from build123d import *

# Parameters (mm, degrees)
SKETCH1_W                                           = 159.95
SKETCH1_H                                           = 159.95
BOSS_EXTRUDE2_DEPTH                                 = 30
SKETCH3_W                                           = 7
SKETCH3_H                                           = 10
BOSS_EXTRUDE4_DEPTH                                 = 145.45
CHAMFER1_SIZE                                       = 0.508
CHAMFER1_SIZE2                                      = 0.03552282
CHAMFER2_SIZE                                       = 0.508
CHAMFER2_SIZE2                                      = 0.03552282
SKETCH4_W                                           = 7.1
SKETCH4_H                                           = 10.2
CUT_EXTRUDE6_DEPTH                                  = 160.2
FILLET1_R                                           = 1
SKETCH6_W                                           = 10.35
SKETCH6_H                                           = 14.5
CUT_EXTRUDE7_DEPTH                                  = 80
BOSS_EXTRUDE5_REACH                                 = 206.773
SKETCH7_W                                           = 14.5
SKETCH7_H                                           = 10.25
CSK_FOR_M4_COUNTERSUNK_FLAT_HEAD_SCREW1_D           = 4.5
CSK_FOR_M4_COUNTERSUNK_FLAT_HEAD_SCREW1_DEPTH       = 16
CSK_FOR_M4_COUNTERSUNK_FLAT_HEAD_SCREW1_CSINK_D     = 9.4
CSK_FOR_M4_COUNTERSUNK_FLAT_HEAD_SCREW1_CSINK_ANGLE = 90
CSK_FOR_M4_COUNTERSUNK_FLAT_HEAD_SCREW1_TIP         = 1.351936393
SKETCH12_R                                          = 2.5
CUT_EXTRUDE9_DEPTH                                  = 5
FILLET2_START                                       = -15.571212121
FILLET2_DEPTH                                       = 154.571212121
FILLET3_START                                       = -15.571212121
FILLET3_DEPTH                                       = 154.571212121
M2_TAPPED_HOLE1_D                                   = 1.6
M2_TAPPED_HOLE1_DEPTH                               = 5.2
M2_TAPPED_HOLE1_TIP                                 = 0.480688495
SKETCH29_W                                          = 20.8
SKETCH29_H                                          = 20.8
SKETCH29_W_2                                        = 12.85
SKETCH29_H_2                                        = 12.85
BOSS_EXTRUDE6_DEPTH                                 = 38
CUT_EXTRUDE15_DEPTH                                 = 207.096620322
CUT_EXTRUDE15_DEPTH_BACK                            = 207.096620322
SKETCH26_W                                          = 10
SKETCH26_H                                          = 10
CUT_EXTRUDE16_DEPTH                                 = 8.5
CUT_EXTRUDE16_DEPTH_BACK                            = 98.4
SKETCH30_W                                          = 10
SKETCH30_H                                          = 10
SKETCH31_W                                          = 12.85
SKETCH31_H                                          = 12.85
CUT_EXTRUDE17_DEPTH                                 = 20
FILLET4_R                                           = 1


with BuildPart() as part:
    # Sketch1 → Boss-Extrude2 (new body)
    with BuildSketch(Plane(origin=(0, 0, 0), x_dir=(1, 0, 0), z_dir=(0, 1, 0))):
        with Locations((57.653787879, -61.85)):
            Rectangle(SKETCH1_W, SKETCH1_H)
    extrude(amount=BOSS_EXTRUDE2_DEPTH)

    # Sketch3 → Boss-Extrude4 (add)
    with BuildSketch(Plane.XY.offset(-18.125)):
        with Locations((141.128787879, 15)):
            Rectangle(SKETCH3_W, SKETCH3_H)
    extrude(amount=BOSS_EXTRUDE4_DEPTH)

    # Chamfer1
    chamfer1_edges = [part.edges().sort_by_distance(p)[0] for p in [
        (144.628787879, 20, 54.6),
    ]]
    chamfer1_side = [part.faces().sort_by_distance(p)[0] for p in [
        (141.128787879, 20, 54.6),
    ]]
    chamfer(chamfer1_edges, length=CHAMFER1_SIZE, length2=CHAMFER1_SIZE2, reference=chamfer1_side[0])

    # Chamfer2
    chamfer2_edges = [part.edges().sort_by_distance(p)[0] for p in [
        (144.628787879, 10, 54.6),
    ]]
    chamfer2_side = [part.faces().sort_by_distance(p)[0] for p in [
        (141.128787879, 10, 54.6),
    ]]
    chamfer(chamfer2_edges, length=CHAMFER2_SIZE, length2=CHAMFER2_SIZE2, reference=chamfer2_side[0])

    # Sketch4 → Cut-Extrude6 (cut)
    with BuildSketch(Plane.ZY.offset(-144.628787879)):
        with Locations((-14.575, 15)):
            Rectangle(SKETCH4_W, SKETCH4_H)
    extrude(amount=CUT_EXTRUDE6_DEPTH, mode=Mode.SUBTRACT)

    # Fillet1
    fillet1_edges = [part.edges().sort_by_distance(p)[0] for p in [
        (144.628787879, 15, -11.025),
    ]]
    fillet(fillet1_edges, radius=FILLET1_R)

    # Sketch6 → Cut-Extrude7 (cut)
    with BuildSketch(Plane(origin=(0, 30, 0), x_dir=(1, 0, 0), z_dir=(0, 1, 0))):
        with Locations((132.453787879, -134.575)):
            Rectangle(SKETCH6_W, SKETCH6_H)
    extrude(amount=-CUT_EXTRUDE7_DEPTH, mode=Mode.SUBTRACT)

    # Boss-Extrude5: up to this face of the body (flat: up to its plane)
    boss_extrude5_end = Plane(part.part.faces().sort_by_distance((57.212424271, 0, 61.420880102))[0])
    # Sketch7 → Boss-Extrude5 (add, up to the picked face)
    with BuildSketch(Plane(origin=(0, 30, 0), x_dir=(1, 0, 0), z_dir=(0, 1, 0)), mode=Mode.PRIVATE) as boss_extrude5_sk1:
        with Locations((-15.071212121, 23.25)):
            Rectangle(SKETCH7_W, SKETCH7_H)
    boss_extrude5_tool1 = split(extrude(boss_extrude5_sk1.sketch, amount=-BOSS_EXTRUDE5_REACH, mode=Mode.PRIVATE), bisect_by=boss_extrude5_end, keep=Keep.BOTH, mode=Mode.PRIVATE)
    add(boss_extrude5_tool1.solids().sort_by(Axis((-15.071212, 30, -23.25), (0, -1, 0)))[0])

    # CSK for M4 Countersunk Flat Head Screw1
    with Locations(Plane.ZY.offset(22.321212121)):
        with Locations((-21, 15)):
            CounterSinkHole(CSK_FOR_M4_COUNTERSUNK_FLAT_HEAD_SCREW1_D / 2, CSK_FOR_M4_COUNTERSUNK_FLAT_HEAD_SCREW1_CSINK_D / 2, depth=CSK_FOR_M4_COUNTERSUNK_FLAT_HEAD_SCREW1_DEPTH, counter_sink_angle=CSK_FOR_M4_COUNTERSUNK_FLAT_HEAD_SCREW1_CSINK_ANGLE)
            with Locations((0, 0, -(CSK_FOR_M4_COUNTERSUNK_FLAT_HEAD_SCREW1_DEPTH + CSK_FOR_M4_COUNTERSUNK_FLAT_HEAD_SCREW1_TIP / 2))):  # 118° drill point
                Cone(0, CSK_FOR_M4_COUNTERSUNK_FLAT_HEAD_SCREW1_D / 2, CSK_FOR_M4_COUNTERSUNK_FLAT_HEAD_SCREW1_TIP, mode=Mode.SUBTRACT)

    # Sketch12 → Cut-Extrude9 (cut)
    with BuildSketch(Plane.XY.offset(127.325)):
        with Locations((132.453787879, 15)):
            Circle(SKETCH12_R)
    extrude(amount=-CUT_EXTRUDE9_DEPTH, mode=Mode.SUBTRACT)

    # Fillet2: read off the stored shape, not the designer's step
    # Fillet2 outline → Fillet2 (cut)
    with BuildSketch(Plane.YZ.offset(FILLET2_START)):
        with BuildLine():
            Line((20.1, -18.125), (21.1, -18.125))
            ThreePointArc((21.1, -18.125), (20.392893219, -17.832106781), (20.1, -17.125))
            Line((20.1, -17.125), (20.1, -18.125))
        make_face()
    extrude(amount=FILLET2_DEPTH, mode=Mode.SUBTRACT)

    # Fillet3: read off the stored shape, not the designer's step
    # Fillet3 outline → Fillet3 (cut)
    with BuildSketch(Plane.YZ.offset(FILLET3_START)):
        with BuildLine():
            ThreePointArc((9.9, -17.125), (9.607106781, -17.832106781), (8.9, -18.125))
            Line((8.9, -18.125), (9.9, -18.125))
            Line((9.9, -18.125), (9.9, -17.125))
        make_face()
    extrude(amount=FILLET3_DEPTH, mode=Mode.SUBTRACT)

    # M2 Tapped Hole1
    with Locations(Plane.XZ):
        with Locations((77.628787879, 41.875)):
            Hole(M2_TAPPED_HOLE1_D / 2, depth=M2_TAPPED_HOLE1_DEPTH)
            with Locations((0, 0, -(M2_TAPPED_HOLE1_DEPTH + M2_TAPPED_HOLE1_TIP / 2))):  # 118° drill point
                Cone(0, M2_TAPPED_HOLE1_D / 2, M2_TAPPED_HOLE1_TIP, mode=Mode.SUBTRACT)

    # Sketch29 → Boss-Extrude6 (add)
    with BuildSketch(Plane(origin=(0, 30, 0), x_dir=(1, 0, 0), z_dir=(0, 1, 0))):
        with Locations((-11.921212121, -131.425)):
            Rectangle(SKETCH29_W, SKETCH29_H)
        with Locations((-11.921212121, -131.425)):
            Rectangle(SKETCH29_W_2, SKETCH29_H_2, mode=Mode.SUBTRACT)
    extrude(amount=BOSS_EXTRUDE6_DEPTH)

    # Sketch26 → Cut-Extrude15 (cut, two sides: drawn at the far end of the back side and taken through both)
    with BuildSketch(Plane(origin=(0, 30, 0), x_dir=(1, 0, 0), z_dir=(0, 1, 0)).offset(-CUT_EXTRUDE15_DEPTH_BACK)):
        with Locations((63.528787879, -55.975)):
            Rectangle(SKETCH26_W, SKETCH26_H)
    extrude(amount=CUT_EXTRUDE15_DEPTH + CUT_EXTRUDE15_DEPTH_BACK, mode=Mode.SUBTRACT)

    # Sketch30 → Cut-Extrude16 (cut, two sides: drawn at the far end of the back side and taken through both)
    with BuildSketch(Plane(origin=(-2.098106061, 0, 2.098106061), x_dir=(-0.7071067811865477, 0, -0.7071067811865475), z_dir=(0.7071067811865475, 0, -0.7071067811865477)).offset(-CUT_EXTRUDE16_DEPTH_BACK)):
        with Locations((-84.501938787, 15)):
            Rectangle(SKETCH30_W, SKETCH30_H)
    extrude(amount=CUT_EXTRUDE16_DEPTH + CUT_EXTRUDE16_DEPTH_BACK, mode=Mode.SUBTRACT)

    # Sketch31 → Cut-Extrude17 (cut)
    with BuildSketch(Plane(origin=(0, 30, 0), x_dir=(1, 0, 0), z_dir=(0, 1, 0))):
        with Locations((-11.921212121, -131.425)):
            Rectangle(SKETCH31_W, SKETCH31_H)
    extrude(amount=-CUT_EXTRUDE17_DEPTH, mode=Mode.SUBTRACT)

    # Fillet4
    fillet4_edges = [part.edges().sort_by_distance(p)[0] for p in [
        (58.528787879, 30, 55.975),
        (63.528787879, 30, 60.975),
        (68.528787879, 30, 55.975),
        (63.528787879, 30, 50.975),
    ]]
    fillet(fillet4_edges, radius=FILLET4_R)


solid = part.part
The listing builds one solid part. Answer for the finished solid, in the listing's coordinates (mm). A direction names the side the tool comes from. Round coordinates to 2 decimals unless told otherwise and drop trailing zeros. Write each loop counter-clockwise with the first axis right and the second up, starting at its lowest first coordinate (ties: lowest second). Pieces come first, ordered by that corner, then holes. Notation, with made-up numbers: M 0,-5 L 59,-5 A20 cw 59,20 Z; hole C 7,7.5 d10. An arc over 180 degrees is marked long. Write each question's results on one line, items separated by ' | '. Start each with the question number.
(1) The part is cut by section B-B, the plane z = -21. Write down the section's boundary in (x, y).
(2) Find the intervals of material crossed by line 1 (X direction, y = 32.5, z = 135); line 2 (Z direction, x = -10, y = 15) (3 decimals); line 3 (Y direction, x = 18, z = -11.5), in increasing order.
(3) The part is cut by section A-A, the plane y = 15. Give the number of separate pieces and of enclosed holes in the cut face, and give its area (3 significant figures).
(4) For faces 4 (the flat face through (-7.821, 15, -24)), 5 (the flat face through (68.529, 14, 56)), 6 (the flat face through (-12, 39, 137.85)), 7 (the flat face through (21, 10, 98)), 8 (the flat face through (136, 15, 127.325)), determine the directions among +Z, -Z, +X, -X, +Y, -Y from which every point of the face is accessible in a straight line to the end or side of a thin tool.
(5) Each of these flat-tipped pins is pushed along its axis until it touches: P1, Ø7, axis at x = 139.5, z = 72.5, coming from the +Y side; P2, Ø4, axis at x = 133.5, y = 15, coming from the +Z side (3 decimals); P3, Ø1.8, axis at x = 74.5, z = -15, coming from the -Y side; P4, Ø1, axis at x = 60.5, y = 16, coming from the -Z side (3 decimals). Where does it stop, or does it pass through?
(6) The part is cut by section D-D, the plane y = 45.5. Write down the section's boundary in (x, z) (3 decimals), and give its area (3 significant figures).
(7) Determine the mould class of faces 1 (the flat face through (29.554, 14.93, 97.021)), 2 (the flat face through (63, 14, 50.975)), 3 (the flat face through (-12.1, 68, 138.2)) for opening direction Y: +Y half, -Y half, draft (parallel to the pull), parting line (faces both ways), or undercut.
(8) The part is cut by section C-C, the plane x = 41. Write down the section's boundary in (y, z) (3 decimals).
Worked answers:
1) outline: M -22.32,0 L -7.82,0 L -7.82,12.75 L -19.87,12.75 L -22.32,10.3 Z; M -22.32,19.7 L -19.87,17.25 L -7.82,17.25 L -7.82,30 L -22.32,30 Z
2) line 1: x = -22.32 to -18.35, -5.5 to -1.52 | line 2: z = -28.375 to -23.25, -18.75 to -18.125, -11.025 to 122.433, 137.85 to 141.825 | line 3: y = 0 to 9.9, 20.1 to 30
3) separate pieces: 2 | enclosed holes: 1 | area: 24,100 mm²
4) face 4: -Z, +X, +Y, -Y | face 5: +Y, -Y | face 6: +Y | face 7: none | face 8: +Z, +X, +Y, -Y
5) P1: stops at y = 30 | P2: stops at z = 127.325 | P3: stops at y = 0 | P4: stops at z = -11.025
6) outline: M -22.321,121.025 L -1.521,121.025 L -1.521,141.825 L -22.321,141.825 Z; hole M -18.346,125 L -5.496,125 L -5.496,137.85 L -18.346,137.85 Z | area: 268 mm²
7) face 1: undercut | face 2: draft | face 3: +Y half
8) outline: M 0,-18.125 L 8.9,-18.125 A1 ccw 9.9,-17.125 L 9.9,-11.025 L 20.1,-11.025 L 20.1,-17.125 A1 ccw 21.1,-18.125 L 30,-18.125 L 30,141.825 L 0,141.825 Z; hole M 10,71.433 L 20,71.433 L 20,85.575 L 10,85.575 Z
